Autodesk Inventor part; units mm, degrees
ref_plane "YZ Plane" through (0, 0, 0) normal (1, 0, 0) x (0, 1, 0)
ref_plane "XZ Plane" through (0, 0, 0) normal (0, 1, 0) x (-1, 0, 0)
ref_plane "XY Plane" through (0, 0, 0) normal (0, 0, 1) x (1, 0, 0)
sketch "StranaDoKotaca" plane through (0, 0, 0) normal (0, 0, 1) x (1, 0, 0)
  arc A0 (10.2, 0) -> (-10.2, 0) centre (0, 0) ccw
  circle A1 centre (-8.2, 0) radius 1
  line L0 (0, 7.2936) -> (0, -4.9994)
  circle A2 centre (8.2, 0) radius 1
  circle A3 centre (0, 0) radius 3.5
  line L1 (-10.2, 0) -> (-13, 0)
  line L2 (10.2, 0) -> (13, 0)
  line L3 (-13, 0) -> (-13, -10.2)
  line L4 (13, 0) -> (13, -10.2)
  line L5 (13, -10.2) -> (-13, -10.2)
  line L6 (0, 10.2) -> (0, 13)
  line L7 (-13, 0) -> (-13, 10.2)
  line L8 (-13, 10.2) -> (13, 10.2)
  line L9 (13, 10.2) -> (13, 0)
  arc A4 (13, 0) -> (8.0598, 10.2) centre (0, 0) ccw
  arc A5 (-8.0598, 10.2) -> (-13, 0) centre (0, 0) ccw
  dimension "d0" = 20.4
  dimension "d4" = 2
  dimension "d5" = 7
  dimension "d6" = 10.2
  dimension "d7" = 10.2
extrude "BocnaStrana" add sketch "StranaDoKotaca" along normal blind 2
sketch "Sketch2" plane through (0, 0, 2) normal (0, 0, 1) x (1, 0, 0)
  arc A0 (10.2, 0) -> (-10.2, 0) centre (0, 0) ccw
  line L0 (-10.2, 0) -> (-10.2, -10.2)
  line L1 (-13, -10.2) -> (13, -10.2)
  line L2 (10.2, 0) -> (10.2, -10.2)
  line L3 (13, 10.2) -> (-13, 10.2)
  line L4 (-13, 10.2) -> (-13, -10.2)
  line L5 (13, -10.2) -> (13, 10.2)
  point P0 (0, 10.2)
  dimension "d12" = 20.4
extrude "Tijelo" add sketch "Sketch2" along normal blind 23 contours A0 L3 L5 L1 L2 | A0 L0 L1 L4 L3
fillet "Rubnik" radius 5 2 edges at (-11.6, -10.2, 25) (11.6, -10.2, 25)
sketch "Sketch3" plane through (-13, 10.2, 0) normal (0, 1, 0) x (1, 0, 0)
  line L0 (26, 0) -> (0, 0)
  line L1 (0, 0) -> (0, -25)
  line L2 (13, -25) -> (0, -25)
  line L3 (13, -2) -> (13, -25)
  line L4 (26, -25) -> (13, -25)
  line L5 (26, 0) -> (26, -25)
  point P0 (13, 0)
extrude "Extrusion3" add sketch "Sketch3" along normal blind 2
properties part number "DrzacZaMotor"
The listing builds one solid part. Answer for the finished solid, in the listing's coordinates (mm). A direction names the side the tool comes from. Coordinates: 2 decimals unless noted, no trailing zeros. Loops run counter-clockwise (first coordinate to the right, second up) from the corner with the lowest first, then second, coordinate; pieces in that order, holes last.
1) Find section B-B on y = 3. Write down the section's boundary in (x, z).
2) Find the intervals of material crossed by L1, parallel to X at y = -7.5, z = 8.25; L2, parallel to Y at x = 8.2, z = 0.45; L3, parallel to Z at x = -6.5, y = -5.5, in increasing order.
3) Determine the mould class of faces 3 (the face through (-7.246, -0.3, 0.986)), 4 (the face through (0, 11, 25)), 5 (the face through (-11.58, -8.7, 23.57)) for opening direction Y: pulls with the +Y half, pulls with the -Y half, needs draft (parallel to the pull), parting line crosses it, or undercut.
4) Find section A-A on x = 0. Write down the section's boundary in (y, z), then the cut area to 3 significant figures.
5) A tool of negligible diameter and unlimited length cuts with its end or side. For faces 1 (the face through (0, 12.2, 12)), 2 (the face through (-0.2, 10.2, 13.3)), from which of +Z, -Z, +X, -X, +Y, -Y can it reach the whole face along a straight path? Write none if from no direction.
6) Find section C-C on z = 14.25. Write down the section's boundary in (x, y).
7) Flat-ended cylindrical pins translate along their axes: pin 1 Ø10 at (x, z) = (1.5, 18) entering from -Y; pin 2 Ø2.5 at (x, y) = (8.2, 0) entering from -Z; pin 3 Ø6 at (x, y) = (4.5, 2.5) entering from +Z; pin 4 Ø5.5 at (x, y) = (0, 0) entering from +Z. Find the tip coordinate at first contact, or state that the pin passes through.
8) Find section D-D on x = -8.2. Write down the section's boundary in (y, z).
Values:
1. outline: (-13, 0) - (-1.8, 0) - (-1.8, 2) - (-9.75, 2) - (-9.75, 25) - (-13, 25) - close; (1.8, 0) - (13, 0) - (13, 25) - (9.75, 25) - (9.75, 2) - (1.8, 2) - close
2. L1: x = -13 to -10.2, 10.2 to 13
2. L2: y = -10.2 to -1, 1 to 12.2
2. L3: z = 0 to 2
3. face 3: undercut
3. face 4: needs draft
3. face 5: pulls with the -Y half
4. outline: (-10.2, 0) - (-3.5, 0) - (-3.5, 2) - (-10.2, 2) - close; (3.5, 0) - (12.2, 0) - (12.2, 25) - (10.2, 25) - (10.2, 2) - (3.5, 2) - close
4. area: 76.8 mm2
5. face 1: +Z, -Z, +X, -X, +Y
5. face 2: +Z, -Y
6. outline: (-13, -10.2) - (-10.2, -10.2) - (-10.2, 0) arc R10.2 cw to (10.2, 0) - (10.2, -10.2) - (13, -10.2) - (13, 12.2) - (-13, 12.2) - close
7. pin 1: stops at y = 7.86
7. pin 2: stops at z = 0
7. pin 3: stops at z = 2
7. pin 4: passes through
8. outline: (-10.2, 0) - (-1, 0) - (-1, 2) - (-10.2, 2) - close; (1, 0) - (12.2, 0) - (12.2, 25) - (6.07, 25) - (6.07, 2) - (1, 2) - close
